The model under review builds one solid part; all positions refer to its coordinate system, in mm. A direction names the side the tool comes from. Coordinates: 2 decimals unless noted, no trailing zeros. Write each loop counter-clockwise with the first axis right and the second up, starting at its lowest first coordinate (ties: lowest second). Pieces come first, ordered by that corner, then holes.
Autodesk Inventor part; units mm, degrees
ref_plane "YZ Plane" through (0, 0, 0) normal (1, 0, 0) x (0, 1, 0)
ref_plane "XZ Plane" through (0, 0, 0) normal (0, 1, 0) x (-1, 0, 0)
ref_plane "XY Plane" through (0, 0, 0) normal (0, 0, 1) x (1, 0, 0)
sketch "Sketch1" plane through (0, 0, 0) normal (1, 0, 0) x (0, 1, 0)
  line L0 (-25, -25) -> (25, -25)
  line L1 (25, -25) -> (25, 25)
  line L2 (25, 25) -> (-25, 25)
  line L3 (-25, 25) -> (-25, -25)
  line L4 (-25, -25) -> (25, 25) construction
  line L5 (25, -25) -> (-25, 25) construction
  line L6 (-24, -24) -> (24, -24)
  line L7 (24, -24) -> (24, 24)
  line L8 (24, 24) -> (-24, 24)
  line L9 (-24, 24) -> (-24, -24)
  line L10 (-24, -24) -> (24, 24) construction
  line L11 (24, -24) -> (-24, 24) construction
  point P0 (0, 0)
  dimension "d0" = 50
  dimension "d1" = 50
  dimension "d2" = 48
  dimension "d3" = 48
extrude "Extrusion1" add sketch "Sketch1" along normal blind 2 contours L3 L2 L1 L0 | L9 L8 L7 L6
sketch "Sketch3" plane through (0, 0, 0) normal (-1, 0, 0) x (0, 0, 1)
  line L0 (19.3, -19.3) -> (-19.3, -19.3)
  line L1 (-19.3, -19.3) -> (-19.3, 19.3)
  line L2 (-19.3, 19.3) -> (19.3, 19.3)
  line L3 (19.3, 19.3) -> (19.3, -19.3)
  line L4 (19.3, -19.3) -> (-19.3, 19.3) construction
  line L5 (-19.3, -19.3) -> (19.3, 19.3) construction
  circle A0 centre (-19.3, 19.3) radius 1.5
  circle A1 centre (19.3, 19.3) radius 1.5555
  circle A2 centre (19.3, -19.3) radius 1.5555
  circle A3 centre (-19.3, -19.3) radius 1.5555
  point P0 (0, 0)
  dimension "d6" = 38.6
  dimension "d7" = 38.6
  dimension "d8" = 3
  dimension "d9" = 3.111
  dimension "d10" = 3.111
  dimension "d11" = 3.111
hole "Hole1" at (0, 19.3, -19.3) direction (1, 0, 0) diameter 3 end through all
sketch "Sketch4" plane through (0, 0, 0) normal (-1, 0, 0) x (0, 0, 1)
  line L0 (-19.3, -19.3) -> (19.3, -19.3)
  line L1 (19.3, -19.3) -> (19.3, 19.3)
  line L2 (19.3, 19.3) -> (-19.3, 19.3)
  line L3 (-19.3, 19.3) -> (-19.3, -19.3)
  line L4 (-19.3, -19.3) -> (19.3, 19.3) construction
  line L5 (19.3, -19.3) -> (-19.3, 19.3) construction
  circle A0 centre (19.3, 19.3) radius 1.5
  point P0 (0, 0)
  dimension "d19" = 38.6
  dimension "d20" = 38.6
  dimension "d21" = 3
hole "Hole2" at (0, 19.3, 19.3) direction (1, 0, 0) diameter 3 end through all
sketch "Sketch5" plane through (0, 0, 0) normal (-1, 0, 0) x (0, 0, 1)
  line L0 (19.3, -19.3) -> (-19.3, -19.3)
  line L1 (-19.3, -19.3) -> (-19.3, 19.3)
  line L2 (-19.3, 19.3) -> (19.3, 19.3)
  line L3 (19.3, 19.3) -> (19.3, -19.3)
  line L4 (19.3, -19.3) -> (-19.3, 19.3) construction
  line L5 (-19.3, -19.3) -> (19.3, 19.3) construction
  circle A0 centre (-19.3, -19.3) radius 1.5
  point P0 (0, 0)
  dimension "d29" = 38.6
  dimension "d30" = 38.6
  dimension "d31" = 3
hole "Hole3" at (0, -19.3, -19.3) direction (1, 0, 0) diameter 3 end through all
sketch "Sketch6" plane through (0, 0, 0) normal (-1, 0, 0) x (0, 0, 1)
  line L0 (19.3, -19.3) -> (-19.3, -19.3)
  line L1 (-19.3, -19.3) -> (-19.3, 19.3)
  line L2 (-19.3, 19.3) -> (19.3, 19.3)
  line L3 (19.3, 19.3) -> (19.3, -19.3)
  line L4 (19.3, -19.3) -> (-19.3, 19.3) construction
  line L5 (-19.3, -19.3) -> (19.3, 19.3) construction
  circle A0 centre (19.3, -19.3) radius 1.5
  point P0 (0, 0)
  dimension "d39" = 38.6
  dimension "d40" = 38.6
  dimension "d41" = 3
hole "Hole4" at (0, -19.3, 19.3) direction (1, 0, 0) diameter 3 end through all
sketch "Sketch7" plane through (0, 0, 0) normal (-1, 0, 0) x (0, 0, 1)
  line L0 (23, -23) -> (-23, -23)
  line L1 (-23, -23) -> (-23, 23)
  line L2 (-23, 23) -> (23, 23)
  line L3 (23, 23) -> (23, -23)
  line L4 (23, -23) -> (-23, 23) construction
  line L5 (-23, -23) -> (23, 23) construction
  line L6 (-25, 25) -> (25, 25)
  line L7 (10, 21) -> (-10, 21)
  line L8 (-10, 21) -> (-10, 25)
  line L9 (-10, 25) -> (10, 25)
  line L10 (10, 25) -> (10, 21)
  line L11 (10, 21) -> (-10, 25) construction
  line L12 (-10, 21) -> (10, 25) construction
  line L13 (21, -10) -> (25, -10)
  line L14 (25, -10) -> (25, 10)
  line L15 (25, 10) -> (21, 10)
  line L16 (21, 10) -> (21, -10)
  line L17 (21, -10) -> (25, 10) construction
  line L18 (25, -10) -> (21, 10) construction
  line L19 (25, -25) -> (-25, -25)
  line L20 (-10, -21) -> (10, -21)
  line L21 (10, -21) -> (10, -25)
  line L22 (10, -25) -> (-10, -25)
  line L23 (-10, -25) -> (-10, -21)
  line L24 (-10, -21) -> (10, -25) construction
  line L25 (10, -21) -> (-10, -25) construction
  line L26 (-25.0252, 10) -> (-20.9748, 10)
  line L27 (-20.9748, 10) -> (-20.9748, -10)
  line L28 (-20.9748, -10) -> (-25.0252, -10)
  line L29 (-25.0252, -10) -> (-25.0252, 10)
  line L30 (-25.0252, 10) -> (-20.9748, -10) construction
  line L31 (-20.9748, 10) -> (-25.0252, -10) construction
  line L32 (25, -25) -> (-25, -25)
  line L33 (-25, -25) -> (-25, 25)
  line L34 (-25, 25) -> (25, 25)
  line L35 (25, 25) -> (25, -25)
  line L36 (25, -25) -> (-25, 25) construction
  line L37 (-25, -25) -> (25, 25) construction
  point P0 (0, 0)
  point P1 (0, 23)
  point P2 (23, 0)
  point P3 (0, -23)
  point P4 (-23, 0)
  point P5 (-10, 23)
  point P6 (10, 23)
  point P7 (23, 10)
  point P8 (23, -10)
  point P9 (10, -23)
  point P10 (-10, -23)
  point P11 (-23, -10)
  point P12 (-23, 10)
  point P13 (10, 25)
  point P14 (-25, 10)
  point P15 (-25, -10)
  point P16 (-10, -25)
  dimension "d49" = 46
  dimension "d50" = 46
  dimension "d51" = 20
  dimension "d52" = 20
  dimension "d53" = 20
  dimension "d54" = 20
extrude "Extrusion3" cut sketch "Sketch7" against normal blind 2 contours L3 L13 L35 L19 L21 L0 | L23 L19 L33 L28 L1 L0 | L3 L2 L10 L6 L35 L15 | L26 L33 L6 L8 L2 L1
sketch "Sketch9" plane through (0, 0, 0) normal (-1, 0, 0) x (0, 0, 1)
  line L0 (10.6, 12.6) -> (-10.6, 12.6)
  line L1 (-12.6, 10.6) -> (-12.6, -10.6)
  line L2 (-10.6, -12.6) -> (10.6, -12.6)
  line L3 (12.6, -10.6) -> (12.6, 10.6)
  line L4 (12.6, 12.6) -> (-12.6, -12.6) construction
  line L5 (-12.6, 12.6) -> (12.6, -12.6) construction
  arc A0 (-12.6, -10.6) -> (-10.6, -12.6) centre (-10.6, -10.6) ccw
  arc A1 (-10.6, 12.6) -> (-12.6, 10.6) centre (-10.6, 10.6) ccw
  arc A2 (12.6, 10.6) -> (10.6, 12.6) centre (10.6, 10.6) ccw
  arc A3 (10.6, -12.6) -> (12.6, -10.6) centre (10.6, -10.6) ccw
  point P0 (0, 0)
  dimension "d62" = 25.2
  dimension "d63" = 25.2
  dimension "d64" = 2
extrude "Extrusion4" cut sketch "Sketch9" against normal blind 2
sketch "Sketch10" plane through (2, 0, 0) normal (1, 0, 0) x (0, 0, -1)
  line L0 (-17, -3) -> (-17, 3) construction
  line L1 (-19, -3) -> (-19, 3)
  line L2 (-15, 3) -> (-15, -3)
  arc A0 (-19, -3) -> (-15, -3) centre (-17, -3) ccw
  arc A1 (-15, 3) -> (-19, 3) centre (-17, 3) ccw
  line L3 (17, -3) -> (17, 3) construction
  line L4 (19, -3) -> (19, 3)
  line L5 (15, 3) -> (15, -3)
  arc A2 (15, -3) -> (19, -3) centre (17, -3) ccw
  arc A3 (19, 3) -> (15, 3) centre (17, 3) ccw
  point P0 (0, 0)
  point P1 (-17, 0)
  point P2 (17, 0)
  dimension "d67" = 17
  dimension "d68" = 17
  dimension "d69" = 4
  dimension "d70" = 4
  dimension "d71" = 10
extrude "Extrusion5" cut sketch "Sketch10" against normal blind 10
fillet "Fillet1" radius 2 4 edges at (1, -23, 23) (1, -23, -23) (1, 23, -23) (1, 23, 23)
properties part number "BottomSide"
Item 1: Take a section at D-D, the plane x = 1.15. Count the separate pieces of the cut face and the enclosed holes in it, plus the area to 3 significant figures.
Solved:
separate pieces: 1
enclosed holes: 7
area: 1,540 mm2
Item 2: Take a section at B-B, the plane z = 17. Write out the cut boundary in (x, y).
Solved:
outline: (0, -23) - (2, -23) - (2, -5) - (0, -5) - close; (0, 5) - (2, 5) - (2, 23) - (0, 23) - close
Item 3: Take a section at A-A, the plane y = 2. Write out the cut boundary in (x, z).
Solved:
outline: (0, -25) - (2, -25) - (2, -19) - (0, -19) - close; (0, -15) - (2, -15) - (2, -12.6) - (0, -12.6) - close; (0, 12.6) - (2, 12.6) - (2, 15) - (0, 15) - close; (0, 19) - (2, 19) - (2, 25) - (0, 25) - close
Item 4: To check wall thickness, follow line 1 along Y through (x, z) = (0.7, -19.3); line 2 along Z through (x, y) = (0.4, 3). State the ranges of each line that lie inside material, in increasing order.
Solved:
line 1: y = -23 to -20.8, -17.8 to 17.8, 20.8 to 23
line 2: z = -25 to -19, -15 to -12.6, 12.6 to 15, 19 to 25
Item 5: Mouldability with a two-part tool opening along Z and no side actions: class faces 1 (the face through (0.99, -12.03, 12)), 2 (the face through (1.01, 22.43, 22.4)), 3 (the face through (1, -10, -24)) as pulls with the +Z half, pulls with the -Z half, needs draft (parallel to the pull), parting line crosses it, or undercut.
Solved:
face 1: undercut
face 2: pulls with the +Z half
face 3: needs draft
Item 6: For pin 1 (0.6 mm diameter, centred on x = 1, z = 14.5, fed in from -Y); pin 2 (0.6 mm diameter, centred on x = 0.5, y = -24, fed in from -Z); pin 3 (1 mm diameter, centred on x = 1.5, y = 13, fed in from -Z), all flat-tipped, find the tip position at first contact; note any pin that passes through.
Solved:
pin 1: stops at y = -23
pin 2: stops at z = -10
pin 3: stops at z = -23
Item 7: Machinability: for faces 4 (the face through (1, 0, -25)), 5 (the face through (1, 23, 15)), 6 (the face through (1, 0, -15)), 7 (the face through (1, -23, 16)), which of the approach directions +Z, -Z, +X, -X, +Y, -Y give a long, thin tool a straight path to every point of the face, cutting with its end or side? Answer none if there is none.
Solved:
face 4: -Z, +X, -X, +Y, -Y
face 5: +Z, +X, -X, +Y
face 6: +X, -X
face 7: +Z, +X, -X, -Y
Item 8: Take a section at C-C, the plane z = -1. Write out the cut boundary in (x, y).
Solved:
outline: (0, -25) - (2, -25) - (2, -12.6) - (0, -12.6) - close; (0, 12.6) - (2, 12.6) - (2, 25) - (0, 25) - close
